from build123d import *

# Parameters (mm, degrees)
SKETCH1_W           = 440
SKETCH1_H           = 310
SKETCH1_R           = 77.5
SKETCH1_R_2         = 1.6
SKETCH1_R_3         = 2
SKETCH1_R_4         = 3
SKETCH1_R_5         = 5
SKETCH1_R_6         = 1.5
SKETCH1_W_2         = 100
SKETCH1_H_2         = 42
SKETCH1_W_3         = 4.605805555
SKETCH1_H_3         = 10.199999311
BOSS_EXTRUDE1_DEPTH = 1.5


with BuildPart() as part:
    # Sketch1 → Boss-Extrude1 (new, symmetric)
    with BuildSketch(Plane(origin=(0, 0, 0), x_dir=(1, 0, 0), z_dir=(0, 1, 0))):
        Rectangle(SKETCH1_W, SKETCH1_H)
        with Locations(Location((0, 0, 0), (0, 0, 270))):
            Circle(SKETCH1_R, mode=Mode.SUBTRACT)
        with Locations(Location((-216.3, 150, 0), (0, 0, 270))):
            Circle(SKETCH1_R_2, mode=Mode.SUBTRACT)
        with Locations(Location((-119.9, 150, 0), (0, 0, 270))):
            Circle(SKETCH1_R_2, mode=Mode.SUBTRACT)
        with Locations(Location((-216.3, 7.5, 0), (0, 0, 270))):
            Circle(SKETCH1_R_2, mode=Mode.SUBTRACT)
        with Locations(Location((-119.9, 7.5, 0), (0, 0, 270))):
            Circle(SKETCH1_R_2, mode=Mode.SUBTRACT)
        with Locations(Location((-216.3, -135.76, 0), (0, 0, 270))):
            Circle(SKETCH1_R_2, mode=Mode.SUBTRACT)
        with Locations(Location((-119.9, -135.76, 0), (0, 0, 270))):
            Circle(SKETCH1_R_2, mode=Mode.SUBTRACT)
        with Locations(Location((214.5, 120, 0), (0, 0, 270))):
            Circle(SKETCH1_R_2, mode=Mode.SUBTRACT)
        with Locations(Location((90.5, 120, 0), (0, 0, 90))):
            Circle(SKETCH1_R_2, mode=Mode.SUBTRACT)
        with Locations(Location((214.5, -69, 0), (0, 0, 90))):
            Circle(SKETCH1_R_2, mode=Mode.SUBTRACT)
        with Locations(Location((90.5, -69, 0), (0, 0, 270))):
            Circle(SKETCH1_R_2, mode=Mode.SUBTRACT)
        with Locations(Location((130.003003206, 30.382091313, 0), (0, 0, 270))):
            Circle(SKETCH1_R_3, mode=Mode.SUBTRACT)
        with Locations(Location((145.003003686, 30.382093295, 0), (0, 0, 270))):
            Circle(SKETCH1_R_3, mode=Mode.SUBTRACT)
        with Locations(Location((160.003004166, 30.382095278, 0), (0, 0, 270))):
            Circle(SKETCH1_R_3, mode=Mode.SUBTRACT)
        with Locations(Location((129.999987649, 15.524988692, 0), (0, 0, 270))):
            Circle(SKETCH1_R_4, mode=Mode.SUBTRACT)
        with Locations(Location((144.999987649, 15.524988692, 0), (0, 0, 270))):
            Circle(SKETCH1_R_4, mode=Mode.SUBTRACT)
        with Locations(Location((159.999987649, 15.524988692, 0), (0, 0, 270))):
            Circle(SKETCH1_R_4, mode=Mode.SUBTRACT)
        with Locations(Location((174.999987649, 15.524988692, 0), (0, 0, 270))):
            Circle(SKETCH1_R_4, mode=Mode.SUBTRACT)
        with Locations(Location((201.839988749, 15.524998187, 0), (0, 0, 270))):
            Circle(SKETCH1_R_5, mode=Mode.SUBTRACT)
        with Locations(Location((214.499987508, 25.52500018, 0), (0, 0, 270))):
            Circle(SKETCH1_R_6, mode=Mode.SUBTRACT)
        with Locations(Location((90.5, 25.5, 0), (0, 0, 270))):
            Circle(SKETCH1_R_6, mode=Mode.SUBTRACT)
        with Locations(Location((129.857092433, -4.478026946, 0), (0, 0, 270))):
            Circle(SKETCH1_R_3, mode=Mode.SUBTRACT)
        with Locations(Location((144.857092433, -4.478026946, 0), (0, 0, 270))):
            Circle(SKETCH1_R_3, mode=Mode.SUBTRACT)
        with Locations(Location((159.857092433, -4.478026946, 0), (0, 0, 270))):
            Circle(SKETCH1_R_3, mode=Mode.SUBTRACT)
        with Locations(Location((174.857092433, -4.478026946, 0), (0, 0, 270))):
            Circle(SKETCH1_R_3, mode=Mode.SUBTRACT)
        with Locations(Location((144.857092433, -19.478026946, 0), (0, 0, 270))):
            Circle(SKETCH1_R_3, mode=Mode.SUBTRACT)
        with Locations(Location((159.857092433, -19.478026946, 0), (0, 0, 270))):
            Circle(SKETCH1_R_3, mode=Mode.SUBTRACT)
        with Locations(Location((174.857092433, -19.478026946, 0), (0, 0, 270))):
            Circle(SKETCH1_R_3, mode=Mode.SUBTRACT)
        with Locations(Location((144.857092433, -34.478026946, 0), (0, 0, 270))):
            Circle(SKETCH1_R_3, mode=Mode.SUBTRACT)
        with Locations(Location((159.857092433, -34.478026946, 0), (0, 0, 270))):
            Circle(SKETCH1_R_3, mode=Mode.SUBTRACT)
        with Locations(Location((174.857092433, -34.478026946, 0), (0, 0, 270))):
            Circle(SKETCH1_R_3, mode=Mode.SUBTRACT)
        with Locations(Location((144.857092433, -49.478026946, 0), (0, 0, 270))):
            Circle(SKETCH1_R_3, mode=Mode.SUBTRACT)
        with Locations(Location((159.857092433, -49.478026946, 0), (0, 0, 270))):
            Circle(SKETCH1_R_3, mode=Mode.SUBTRACT)
        with Locations(Location((174.857092433, -49.478026946, 0), (0, 0, 270))):
            Circle(SKETCH1_R_3, mode=Mode.SUBTRACT)
        with Locations(Location((129.857092433, -19.478026946, 0), (0, 0, 270))):
            Circle(SKETCH1_R_3, mode=Mode.SUBTRACT)
        with Locations(Location((129.857092433, -34.478026946, 0), (0, 0, 270))):
            Circle(SKETCH1_R_3, mode=Mode.SUBTRACT)
        with Locations(Location((129.857092433, -49.478026946, 0), (0, 0, 270))):
            Circle(SKETCH1_R_3, mode=Mode.SUBTRACT)
        with Locations((152.5, 82.7)):
            Rectangle(SKETCH1_W_2, SKETCH1_H_2, mode=Mode.SUBTRACT)
        with Locations((214.933136209, 82.091000898)):
            Rectangle(SKETCH1_W_3, SKETCH1_H_3, mode=Mode.SUBTRACT)
    extrude(amount=BOSS_EXTRUDE1_DEPTH, both=True)


solid = part.part
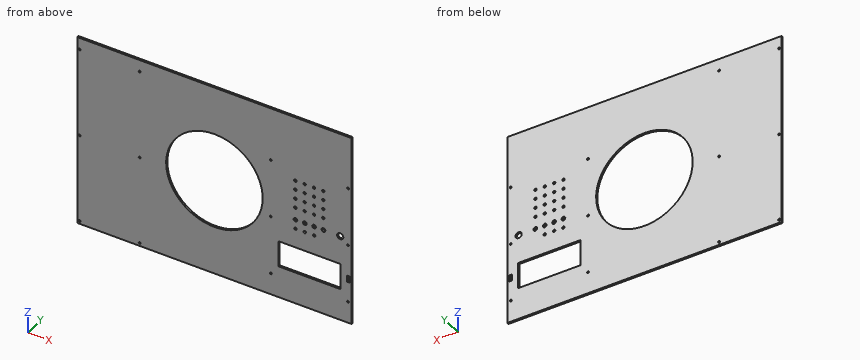
Geometry check sheet. Reference: the model listing, model coordinates, mm. Coordinates: 2 decimals unless noted, no trailing zeros. Order: outer loops, then holes, each group sorted by start corner. A loop starts at its lowest first (then second) coordinate and runs counter-clockwise, first axis right, second up. Notation, with made-up numbers: (-12.5, 59.25) - (20.5, 59.25) arc R17 cw to (20.5, 85.25) - close; hole circle Ø11 at (86, -5). An arc over 180 degrees is marked (long way). Answer in a Markdown table with one row per item. Add a question column.
1) Cross-section at A-A, the plane x = 60. Record the cut outline in (y, z), then the cut area to 3 significant figures.
2) Material ranges on line 1 along Z through (x, y) = (-119.9, 0.05); line 2 along X through (y, z) = (-0.6, -25.5); line 3 along X through (y, z) = (0.7, -2), recorded low to high. Write a range as [from, to].
3) Cross-section at B-B, the plane x = 186.5. Record the cut outline in (y, z).
4) Cross-section at C-C, the plane y = 0.2. State how many separate pieces and enclosed holes the cut face has, then the cut area to 3 significant figures.
5) Gauge pin test, flat end, axial feed: P1, Ø4, axis at x = -25.5, z = 70, coming from the +Y side. Record the tip position at first contact, or that the pin passes through.
Check result:
| question | item | result |
|---|---|---|
| 1 | outline | (-1.5, -155) - (1.5, -155) - (1.5, -49.05) - (-1.5, -49.05) - close; (-1.5, 49.05) - (1.5, 49.05) - (1.5, 155) - (-1.5, 155) - close |
| 1 | area | 636 mm² |
| 2 | line 1 | z = [-155, -151.6], [-148.4, -9.1], [-5.9, 134.16], [137.36, 155] |
| 2 | line 2 | x = [-220, -73.18], [73.18, 89], [92, 213], [216, 220] |
| 2 | line 3 | x = [-220, -77.47], [77.47, 220] |
| 3 | outline | (-1.5, -155) - (1.5, -155) - (1.5, -103.7) - (-1.5, -103.7) - close; (-1.5, -61.7) - (1.5, -61.7) - (1.5, 155) - (-1.5, 155) - close |
| 4 | separate pieces | 1 |
| 4 | enclosed holes | 39 |
| 4 | area | 113,000 mm² |
| 5 | P1 | passes through |
